Job drawing, mm, ordinate dimensions from the low corner. One solid piece. Round coordinates to 2 decimals unless told otherwise and drop trailing zeros. Loops run counter-clockwise (first coordinate to the right, second up) from the corner with the lowest first, then second, coordinate; pieces in that order, holes last. Notation, with made-up numbers: M 51.25,-39 L 102.25,-39 A23 cw 102.25,-8 Z; hole C 75.25,-17.5 d11. An arc over 180 degrees is marked long. Use a Markdown table: item, result. Add a question column.
(1) Two-plate mould, pull along Y, no slides. Class the marked faces 1, 2 and 3: released by +Y, released by -Y, zero draft, split by the parting line, or undercut.
(2) Band-saw the part on A-A, the plane x = 10.16. Give the number of separate pieces and of enclosed holes in the cut face.
(3) Band-saw the part on C-C, the plane z = 5.5. Write the cut outline in (x, y) (1 decimal).
(4) Wall check: L1, parallel to Y at x = 10.16, z = 6; L2, parallel to Y at x = 10.16, z = 2.5; L3, parallel to Y at x = 7.75, z = 6.75 (1 decimal). Give the ranges that are in metal, low to high.
(5) Band-saw the part on B-B, the plane y = 10.16. Write the cut outline in (x, z).
(6) Flat gauge pins, fed straight in: P1, Ø8, axis at x = 10.16, y = 10.16, coming from the -Z side; P2, Ø1, axis at x = 14.5, z = 5.5, coming from the -Y side; P3, Ø3, axis at y = 16, z = 5, coming from the +X side. Where does each tip first touch, or does it go through?
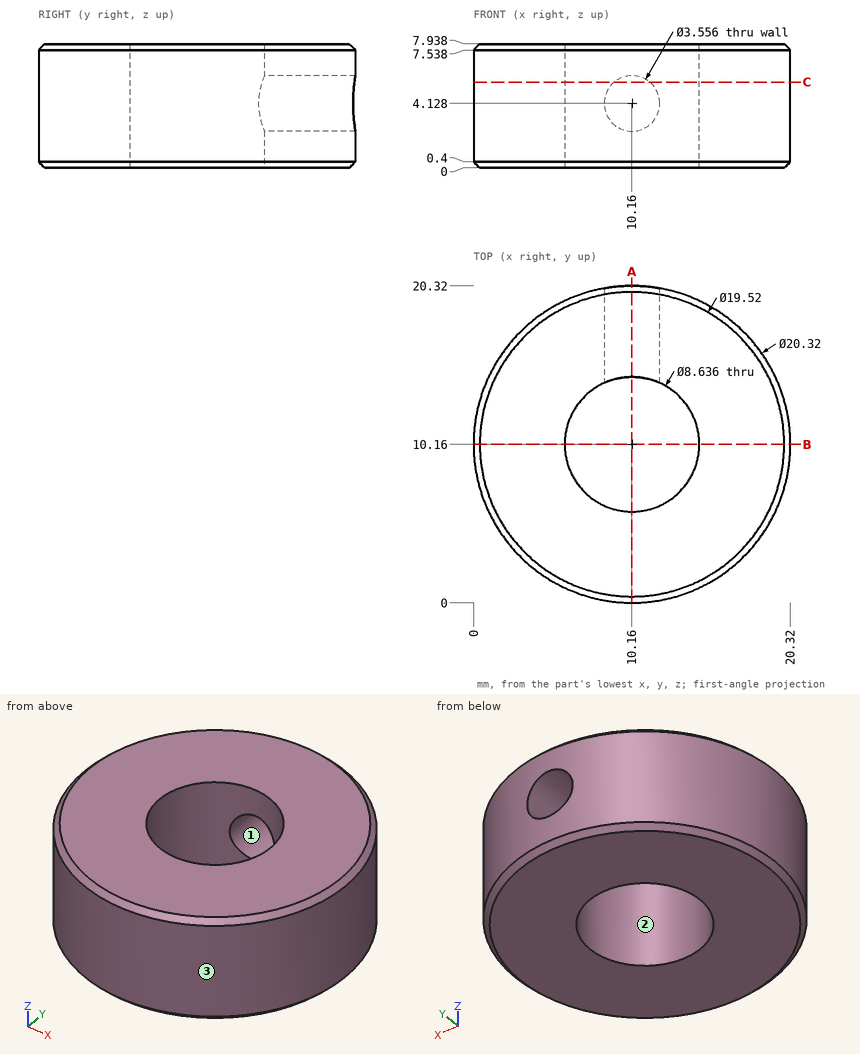
Return value:
| question | item | result |
|---|---|---|
| 1 | face 1 | zero draft |
| 1 | face 2 | undercut |
| 1 | face 3 | split by the parting line |
| 2 | separate pieces | 3 |
| 2 | enclosed holes | 0 |
| 3 | outline | M 9,14.3 L 9,20.3 A10.2 ccw long 11.3,20.3 L 11.3,14.3 A4.3 cw long Z |
| 4 | L1 | 0 to 5.84, 14.48 to 20.32 |
| 4 | L2 | 0 to 5.84 |
| 4 | L3 | 0.3 to 6.6, 13.7 to 20 |
| 5 | outline | M 0,0.4 L 0.4,0 L 5.84,0 L 5.84,7.94 L 0.4,7.94 L 0,7.54 Z; M 14.48,0 L 19.92,0 L 20.32,0.4 L 20.32,7.54 L 19.92,7.94 L 14.48,7.94 Z |
| 6 | P1 | through |
| 6 | P2 | y = 0.75 |
| 6 | P3 | x = 19.35 |
